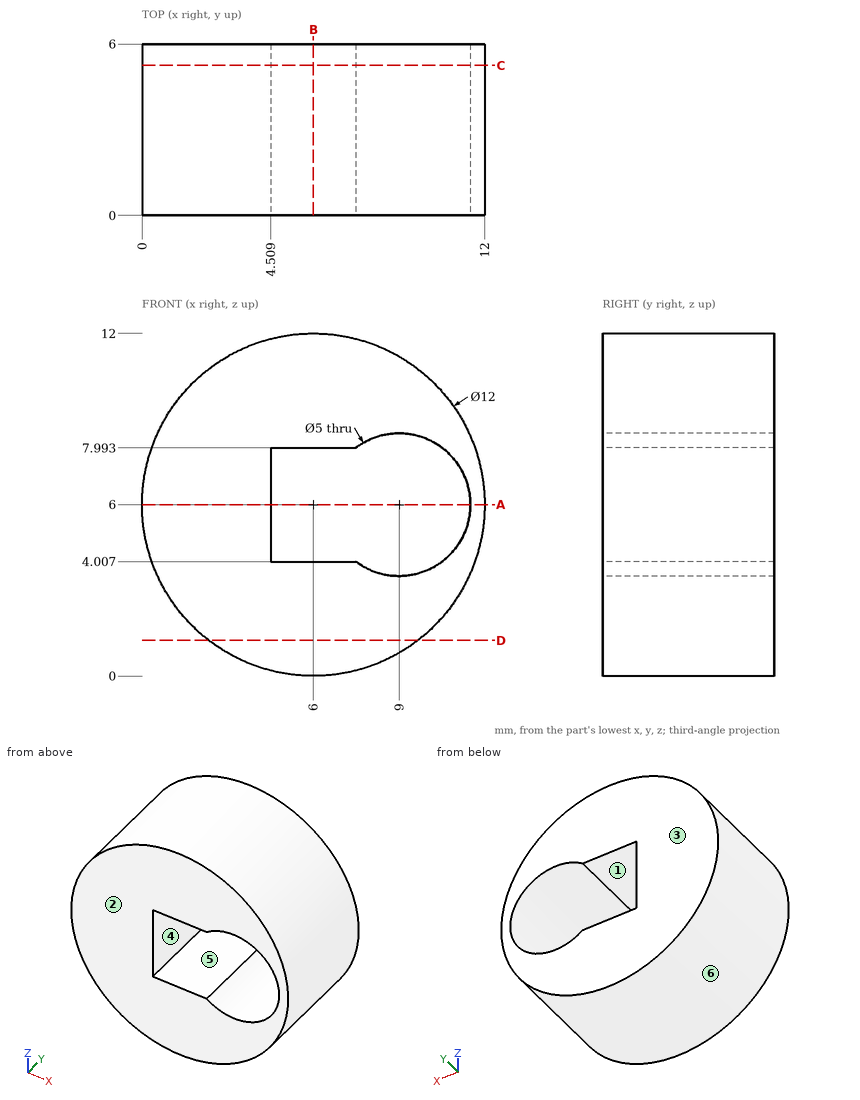
Geometry check sheet. Reference: drawing and pictorial views, mm from the part's lowest x, y, z. A direction names the side the tool comes from. Coordinates: 2 decimals unless noted, no trailing zeros. Loops run counter-clockwise (first coordinate to the right, second up) from the corner with the lowest first, then second, coordinate; pieces in that order, holes last. Notation, with made-up numbers: M 82,-27.5 L 123,-27.5 A6 cw 123,-22.5 Z; hole C 67,-4.5 d9. An arc over 180 degrees is marked long. One line per item, written item: value.
1. Material ranges on line 1 along X through (y, z) = (2.3, 6); line 2 along Z through (x, y) = (9.75, 1.8) (1 decimal); line 3 along X through (y, z) = (1.05, 6.5), recorded low to high. Write a range as from..to.
Answers follow:
line 1: 0..4.51, 11.5..12
line 2: 1.3..3.6, 8.4..10.7
line 3: 0.02..4.51, 11.45..11.98
2. Section check A-A on z = 6. Record the cut outline in (x, y).
Answers follow:
outline: M 0,0 L 4.51,0 L 4.51,6 L 0,6 Z; M 11.5,0 L 12,0 L 12,6 L 11.5,6 Z
3. Set-up check for the marked faces 1 and 2: record each of +Z, -Z, +X, -X, +Y, -Y from which the full face is reachable in a straight line by a thin tool's end or side.
Answers follow:
face 1: +Y, -Y
face 2: +Z, -Z, +X, -X, -Y
4. Section check C-C on y = 5.25. Record the cut outline in (x, z).
Answers follow:
outline: C 6,6 d12; hole M 4.51,4.01 L 7.49,4.01 A2.5 ccw long 7.49,7.99 L 4.51,7.99 Z
5. Section check B-B on x = 6. Record the cut outline in (y, z).
Answers follow:
outline: M 0,0 L 6,0 L 6,4.01 L 0,4.01 Z; M 0,7.99 L 6,7.99 L 6,12 L 0,12 Z
6. Mould release check, pull along Z, two halves, no side actions. Record for the marked faces 3, 4, 5 and 6: pulls with the +Z half, pulls with the -Z half, needs draft (parallel to the pull), parting line crosses it, or undercut.
Answers follow:
face 3: needs draft
face 4: undercut
face 5: undercut
face 6: parting line crosses it
7. Gauge pin test, flat ends, axial feed: P1, Ø1, axis at x = 6, z = 2.5, coming from the -Y side; P2, Ø4, axis at x = 9, z = 6, coming from the +Y side; P3, Ø3, axis at y = 5, z = 4, coming from the -X side; P4, Ø3, axis at x = 3, y = 3.5, coming from the -Z side. Record the tip position at first contact, or that the pin passes through.
Answers follow:
P1: y = 0
P2: through
P3: x = 0.02
P4: z = 0.19
8. Section check D-D on z = 1.25. Record the cut outline in (x, y), plus the area to 3 significant figures.
Answers follow:
outline: M 2.33,0 L 9.67,0 L 9.67,6 L 2.33,6 Z
area: 44.0 mm^2
